Model file for the job. Use its own axes, mm. Coordinates: 2 decimals unless noted, no trailing zeros. Loops run counter-clockwise (first coordinate to the right, second up) from the corner with the lowest first, then second, coordinate; pieces in that order, holes last.
Autodesk Fusion 360 part; units mm, degrees
sketch "Sketch1" plane through (0, 0, 0) normal (0, 0, 1) x (1, 0, 0)
  line L0 (0, 0) -> (100, 0)
  line L1 (100, 0) -> (100, -150)
  line L2 (0, 0) -> (0, -150)
  line L3 (0, -150) -> (100, -150)
  dimension "d1" = 100
  dimension "d2" = 150
extrude "Extrude1" add sketch "Sketch1" along normal blind 5
hole "Hole1" at (10, -10, 5) direction (0, 0, -1) diameter 10 depth 5 tip angle 180
hole "Hole2" at (90, -10, 5) direction (0, 0, -1) diameter 10 depth 5 tip angle 180
hole "Hole3" at (10, -140, 5) direction (0, 0, -1) diameter 10 depth 5 tip angle 180
hole "Hole4" at (90, -140, 5) direction (0, 0, -1) diameter 10 depth 5 tip angle 180
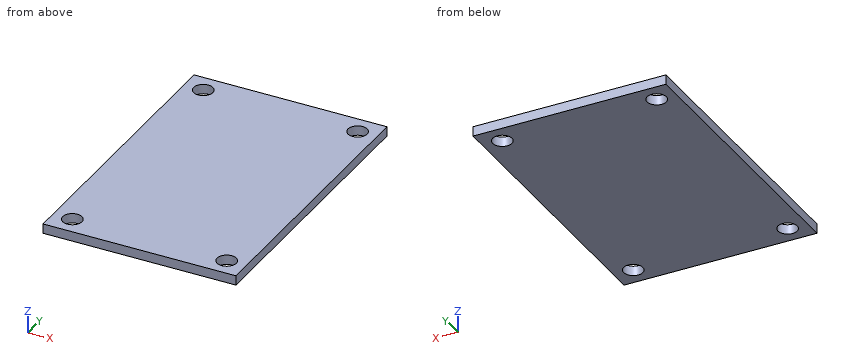
Q1. Slice it at B-B (x = 90). List the corners of the cut face in (y, z), and give its area (3 significant figures).
Answers:
outline: (-150, 0) - (-145, 0) - (-145, 5) - (-150, 5) - close; (-135, 0) - (-15, 0) - (-15, 5) - (-135, 5) - close; (-5, 0) - (0, 0) - (0, 5) - (-5, 5) - close
area: 650 mm2
Q2. Slice it at A-A (y = -140). List the corners of the cut face in (x, z).
Answers:
outline: (0, 0) - (5, 0) - (5, 5) - (0, 5) - close; (15, 0) - (85, 0) - (85, 5) - (15, 5) - close; (95, 0) - (100, 0) - (100, 5) - (95, 5) - close
Q3. Slice it at C-C (z = 3.4). List the corners of the cut face in (x, y).
Answers:
outline: (0, -150) - (100, -150) - (100, 0) - (0, 0) - close; hole circle Ø10 at (10, -140); hole circle Ø10 at (10, -10); hole circle Ø10 at (90, -140); hole circle Ø10 at (90, -10)
Q4. Drill centre lines: line 1 (X direction, y = -140, z = 3.7); line 2 (Y direction, x = 10, z = 2.5); line 3 (Y direction, x = 11, z = 3). Where is each one in solid material? Low to high.
Answers:
line 1: x = 0 to 5, 15 to 85, 95 to 100
line 2: y = -150 to -145, -135 to -15, -5 to 0
line 3: y = -150 to -144.9, -135.1 to -14.9, -5.1 to 0
